Input: part model. Units: mm. Frame: model coordinates. Face numbers are marked on the shaded views. A direction names the side the tool comes from. Coordinates: 2 decimals unless noted, no trailing zeros. Order: outer loops, then holes, each group sorted by start corner. A loop starts at its lowest first (then second) coordinate and runs counter-clockwise, first axis right, second up. Notation, with made-up numbers: (7, 50.5) -> (25, 50.5) arc R14 cw to (25, 63.5) -> close; hole circle Ø2 at (-19, 50). An arc over 180 degrees is marked (long way). Answer as CSV lines item,"result".
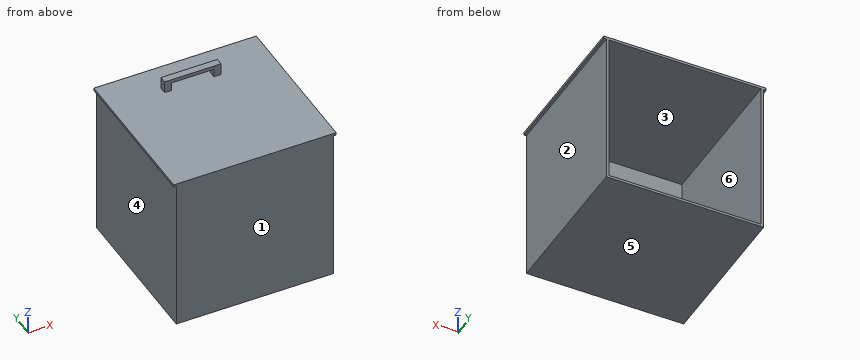
from build123d import *

# Parameters (mm, degrees)
BOSS_EXTRUDE1_DEPTH = 550
SKETCH3_W           = 540
SKETCH3_H           = 546
CUT_EXTRUDE1_DEPTH  = 545
SKETCH4_W           = 200
SKETCH4_H           = 25
BOSS_EXTRUDE2_DEPTH = 43
SKETCH6_W           = 150
SKETCH6_H           = 30
CUT_EXTRUDE2_DEPTH  = 25


with BuildPart() as part:
    # Sketch1 → Boss-Extrude1 (new body)
    with BuildSketch(Plane(origin=(0, 0, 0), x_dir=(1, 0, 0), z_dir=(0, 1, 0))):
        Polygon((-382.12099403, -271.280172414), (-373.12099403, -271.280172414), (-373.12099403, 283.719827586), (184.87900597, 283.719827586), (184.87900597, -271.280172414), (193.87900597, -271.280172414), (193.87900597, -280.280172414), (-382.12099403, -280.280172414), align=None)
    extrude(amount=BOSS_EXTRUDE1_DEPTH)

    # Sketch3 → Cut-Extrude1 (cut)
    with BuildSketch(Plane(origin=(0, 550, 0), x_dir=(1, 0, 0), z_dir=(0, 1, 0))):
        with Locations((-94.12099403, 1.719827586)):
            Rectangle(SKETCH3_W, SKETCH3_H)
    extrude(amount=-CUT_EXTRUDE1_DEPTH, mode=Mode.SUBTRACT)

    # Sketch4 → Boss-Extrude2 (add)
    with BuildSketch(Plane.XY.offset(280.280172414)):
        with Locations((-94.12099403, 440.468229794)):
            Rectangle(SKETCH4_W, SKETCH4_H)
    extrude(amount=BOSS_EXTRUDE2_DEPTH)

    # Sketch6 → Cut-Extrude2 (cut)
    with BuildSketch(Plane(origin=(0, 452.968229794, 0), x_dir=(1, 0, 0), z_dir=(0, 1, 0))):
        with Locations((-94.12099403, -295.280172414)):
            Rectangle(SKETCH6_W, SKETCH6_H)
    extrude(amount=-CUT_EXTRUDE2_DEPTH, mode=Mode.SUBTRACT)


solid = part.part
1. Cut plane C-C (y = 47). Return the cut outline in (x, z), plus the area to 3 significant figures.
Findings:
outline,"(-382.12, 271.28) -> (-373.12, 271.28) -> (-373.12, -283.72) -> (184.88, -283.72) -> (184.88, 271.28) -> (193.88, 271.28) -> (193.88, 280.28) -> (-382.12, 280.28) -> close; hole (-364.12, -274.72) -> (175.88, -274.72) -> (175.88, 271.28) -> (-364.12, 271.28) -> close"
area,"20,000 mm2"
2. Cut plane B-B (y = 444). Return the cut outline in (x, z), plus the area to 3 significant figures.
Findings:
outline,"(-382.12, 271.28) -> (-373.12, 271.28) -> (-373.12, -283.72) -> (184.88, -283.72) -> (184.88, 271.28) -> (193.88, 271.28) -> (193.88, 280.28) -> (5.88, 280.28) -> (5.88, 323.28) -> (-194.12, 323.28) -> (-194.12, 280.28) -> (-382.12, 280.28) -> close; hole (-364.12, -274.72) -> (175.88, -274.72) -> (175.88, 271.28) -> (-364.12, 271.28) -> close; hole (-169.12, 280.28) -> (-19.12, 280.28) -> (-19.12, 310.28) -> (-169.12, 310.28) -> close"
area,"24,100 mm2"
3. Cut plane D-D (x = -331.5). Return the cut outline in (y, z), plus the area to 3 significant figures.
Findings:
outline,"(0, -283.72) -> (550, -283.72) -> (550, -274.72) -> (5, -274.72) -> (5, 271.28) -> (550, 271.28) -> (550, 280.28) -> (0, 280.28) -> close"
area,"12,600 mm2"
4. Ray query, line 1 along Z through (x, y) = (24.5, 265); line 2 along X through (y, z) = (113, -66.5); line 3 along Y through (x, z) = (-232, 201.5). Return the intervals inside material, ascending.
Findings:
line 1,"z = -283.72 to -274.72, 271.28 to 280.28"
line 2,"x = -373.12 to -364.12, 175.88 to 184.88"
line 3,"y = 0 to 5"
5. Contact query for flat-ended pins moving along their axis: pin 1 (3 mm diameter, centred on x = 110, y = 329, fed in from +Z); pin 2 (12.5 mm diameter, centred on y = 436.5, z = 302, fed in from -X); pin 3 (10 mm diameter, centred on y = 307, z = 128, fed in from +X); pin 4 (13 mm diameter, centred on x = -92, z = 293, fed in from -Y). Output: stop coordinate, or through.
Findings:
pin 1,"stops at z = 280.28"
pin 2,"stops at x = -194.12"
pin 3,"stops at x = 184.88"
pin 4,"passes through"
6. Mould query, pull axis Z, two halves, no side actions, for the marked faces 4, 5 and 6. Classes: released by +Z, released by -Z, zero draft, split by the parting line, or undercut.
Findings:
face 4,"zero draft"
face 5,"released by -Z"
face 6,"undercut"
7. Reachability of the marked faces 1, 2 and 3 from +Z, -Z, +X, -X, +Y, -Y: full face, straight path, thin tool, end or side. Return the list, or none.
Findings:
face 1,"+Z, -Z, +X, -X, -Y"
face 2,"-Z, +X, +Y, -Y"
face 3,"+Y"
8. Cut plane A-A (x = -153). Return the cut outline in (y, z).
Findings:
outline,"(0, -283.72) -> (550, -283.72) -> (550, -274.72) -> (5, -274.72) -> (5, 271.28) -> (550, 271.28) -> (550, 280.28) -> (0, 280.28) -> close; (427.97, 310.28) -> (452.97, 310.28) -> (452.97, 323.28) -> (427.97, 323.28) -> close"
